Could you check a few things on this model? Use its own coordinates, in mm. Face numbers are marked on the shaded views. Give positions to 0.01 mm unless a question says otherwise; leave off trailing zeros. Loops run counter-clockwise (first coordinate to the right, second up) from the corner with the lowest first, then second, coordinate; pieces in that order, holes last. Notation, with made-up numbers: M -22.75,-4 L 29.25,-4 A18 cw 29.25,17 Z; hole C 49.25,-33 d8. An arc over 180 degrees is marked long. Answer in a Markdown table with one row per item. Add a question column.
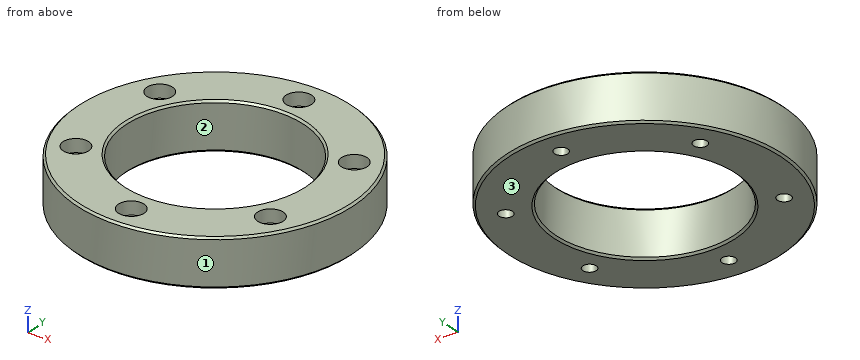
```python
from build123d import *

# Parameters (mm, degrees)
SKETCH_1_R                   = 35
SKETCH_1_R_2                 = 22.5
EXTRUDE_1_DEPTH              = 6
HOLE_WIZARD_M3_1_D           = 3.4
HOLE_WIZARD_M3_1_CBORE_D     = 6.5
HOLE_WIZARD_M3_1_CBORE_DEPTH = 3.3
PATTERN_CIRCULAR_1_COUNT     = 6
CHAMFER_1_SIZE               = 0.5


with BuildPart() as part:
    # Sketch 1 → Extrude 1 (new, symmetric)
    with BuildSketch(Plane.XY):
        Circle(SKETCH_1_R)
        Circle(SKETCH_1_R_2, mode=Mode.SUBTRACT)
    extrude(amount=EXTRUDE_1_DEPTH, both=True)

    # Hole Wizard M3 _ _ _ _ _ _1 (through all)
    with Locations(Plane.XY.offset(6)):
        with Locations((0, 28.5)):
            hole_wizard_m3_1 = CounterBoreHole(HOLE_WIZARD_M3_1_D / 2, HOLE_WIZARD_M3_1_CBORE_D / 2, HOLE_WIZARD_M3_1_CBORE_DEPTH)

    # Pattern Circular 1: Hole Wizard M3 _ _ _ _ _ _1 ×6 about axis
    pattern_circular_1_axis = Axis((0, 0, 0), (0, 0, 1))
    for i in range(1, PATTERN_CIRCULAR_1_COUNT):
        add(hole_wizard_m3_1.rotate(pattern_circular_1_axis, i * 360 / PATTERN_CIRCULAR_1_COUNT), mode=Mode.SUBTRACT)

    # Chamfer 1
    chamfer_1_edges = [part.edges().sort_by_distance(p)[0] for p in [
        (-35, 0, -6),
        (-35, 0, 6),
        (-22.5, 0, -6),
        (-22.5, 0, 6),
    ]]
    chamfer(chamfer_1_edges, length=CHAMFER_1_SIZE)


solid = part.part
```
Item 1: Suppose I cut it at B-B (y = 0). List the corners of the cut face in (x, z) for me.
Item 2: For P1, Ø3, axis at x = -23.5, y = -13.5, coming from the +Z side; P2, Ø5, axis at x = -12, z = -4.5, coming from the -Y side; P3, Ø2.5, axis at x = -24.68, y = -14.25, coming from the +Z side; P4, Ø1.5, axis at x = 27.5, z = 4.5, coming from the +Y side, each with a flat end and sliding along its axis, tell me the tip position at first contact or that it passes through.
Item 3: If we mould it in two halves opening along Y, with no side actions, what happens to the marked faces 1, 2 and 3? For each: +Y half, -Y half, draft (parallel to the pull), parting line (faces both ways), or undercut.
Item 4: Suppose I cut it at A-A (x = 0). Give the number of separate pieces and of enclosed holes in the cut face, then the cut area to 3 significant figures.
Item 5: I need wall thicknesses on L1, parallel to X at y = 12.5, z = 3.5; L2, parallel to Y at x = -1.5, z = 4.75; L3, parallel to X at y = 10.5, z = 0. Which ranges of each line are inside material? Lowest first, please.
Values found:
| question | item | result |
|---|---|---|
| 1 | outline | M -35,-5.5 L -34.5,-6 L -23,-6 L -22.5,-5.5 L -22.5,5.5 L -23,6 L -34.5,6 L -35,5.5 Z; M 22.5,-5.5 L 23,-6 L 34.5,-6 L 35,-5.5 L 35,5.5 L 34.5,6 L 23,6 L 22.5,5.5 Z |
| 2 | P1 | z = 2.7 |
| 2 | P2 | y = -33.69 |
| 2 | P3 | through |
| 2 | P4 | y = 22.57 |
| 3 | face 1 | parting line |
| 3 | face 2 | undercut |
| 3 | face 3 | draft |
| 4 | separate pieces | 4 |
| 4 | enclosed holes | 0 |
| 4 | area | 197 mm² |
| 5 | L1 | -32.69 to -27.42, -21.94 to -18.71, 18.71 to 21.94, 27.42 to 32.69 |
| 5 | L2 | -34.97 to -31.38, -25.62 to -22.45, 22.45 to 25.62, 31.38 to 34.97 |
| 5 | L3 | -33.39 to -19.9, 19.9 to 33.39 |
